Autodesk Inventor part; units mm, degrees
ref_plane "YZ Plane" through (0, 0, 0) normal (1, 0, 0) x (0, 1, 0)
ref_plane "XZ Plane" through (0, 0, 0) normal (0, 1, 0) x (-1, 0, 0)
ref_plane "XY Plane" through (0, 0, 0) normal (0, 0, 1) x (1, 0, 0)
sketch "Sketch1" plane through (0, 0, 0) normal (0, 0, 1) x (1, 0, 0)
  line L0 (-7, 7) -> (7, 7)
  line L1 (7, 7) -> (7, -7)
  line L2 (7, -7) -> (-7, -7)
  line L3 (-7, -7) -> (-7, 7)
  line L4 (-7, 7) -> (7, -7) construction
  line L5 (7, 7) -> (-7, -7) construction
  point P0 (0, 0)
  dimension "d0" = 14
  dimension "d1" = 14
extrude "Extrusion1" add sketch "Sketch1" along normal blind 28
sketch "Sketch2" plane through (7, -7, 0) normal (1, 0, 0) x (0, 0, -1)
  line L0 (-28, 0) -> (-28, 14)
  line L1 (-28, 14) -> (-14, 14)
  line L2 (-14, 14) -> (-14, 0)
  line L3 (-14, 0) -> (-28, 0)
  line L4 (-28, 0) -> (-28, 14)
  point P0 (0, 7)
  dimension "d4" = 14
  dimension "d5" = 14
extrude "Extrusion2" add sketch "Sketch2" along normal blind 14
sketch "Sketch3" plane through (21, -7, 0) normal (1, 0, 0) x (0, 0, -1)
  line L0 (-14, 0) -> (-14, 14)
  line L1 (-14, 14) -> (-28, 14)
  line L2 (-28, 14) -> (-28, 0)
  line L3 (-28, 0) -> (-14, 0)
  line L4 (-28, 14) -> (-14, 14)
  line L5 (-14, 14) -> (-14, 0)
  line L6 (-14, 0) -> (-28, 0)
  line L7 (-28, 0) -> (-28, 14)
  point P0 (0, 7)
  point P1 (-21, 7)
hole "Hole1" at (21, 0, 21) direction (-1, 0, 0) diameter 8 depth 25
sketch "Sketch4" plane through (0, 0, 0) normal (0, 0, -1) x (-1, 0, 0)
  line L0 (7, -7) -> (-7, -7)
  line L1 (7, 7) -> (7, -7)
  line L2 (-7, 7) -> (7, 7)
  line L3 (-7, -7) -> (-7, 7)
  point P0 (0, 0)
  point P1 (0, 0)
sketch "Sketch5" plane through (-7, 7, 0) normal (0, 1, 0) x (1, 0, 0)
  line L0 (14, 0) -> (0, 0)
  line L1 (0, 0) -> (0, -28)
  line L2 (0, -28) -> (28, -28)
  line L3 (28, -14) -> (28, -28)
  line L4 (14, -14) -> (28, -14)
  line L5 (14, 0) -> (14, -14)
  line L6 (14, -14) -> (28, -14)
  line L7 (28, -14) -> (28, -28)
  line L8 (28, -28) -> (14, -28)
  line L9 (14, -28) -> (14, -14)
  circle A0 centre (21, -21) radius 4
  point P0 (7, 0)
  dimension "d23" = 8
extrude "Extrusion3" add sketch "Sketch5" along normal blind 45 contours A0
thread "Thread1"
sketch "Sketch6" plane through (14, 52, 21) normal (0, 1, 0) x (1, 0, 0)
  circle A0 centre (0, 0) radius 4
  point P0 (-14, 21)
hole "Hole3" at (14, 52, 21) direction (0, -1, 0) diameter 6 depth 50 tip angle 118
sketch "Sketch7" plane through (-7, -7, 0) normal (0, -1, 0) x (1, 0, 0)
  line L0 (28, 28) -> (28, 14)
  line L1 (14, 14) -> (28, 14)
  line L2 (28, 28) -> (14, 28)
  line L3 (14, 28) -> (14, 14)
  line L4 (14, 14) -> (28, 14)
  line L5 (28, 14) -> (28, 28)
  circle A0 centre (21, 21) radius 3
  circle A1 centre (21, 21) radius 7
  circle A2 centre (21, 21) radius 4
  circle A3 centre (21, 21) radius 4
  line L6 (21, 21) -> (0, 21)
  line L7 (0, 0) -> (0, 28)
  line L8 (0, 21) -> (0, 34.5)
  line L9 (0, 34.5) -> (0, 21)
  line L10 (0, 21) -> (0, 7.5)
  point P0 (7, 0)
  dimension "d35" = 14
  dimension "d36" = 8
  dimension "d37" = 13.5
  dimension "d38" = 13.5
sketch "Sketch8" plane through (0, 0, 0) normal (0, 0, -1) x (-1, 0, 0)
  line L0 (7, -7) -> (-7, -7)
  line L1 (7, 7) -> (7, -7)
  line L2 (-7, -7) -> (7, -7)
  line L3 (7, -7) -> (7, 7)
  line L4 (7, 7) -> (-7, 7)
  line L5 (-7, 7) -> (-7, -7)
  point P0 (0, 0)
extrude "Extrusion4" cut sketch "Sketch8" against normal blind 7.5
sketch "Sketch9" plane through (0, 0, 28) normal (0, 0, 1) x (1, 0, 0)
  line L0 (-7, 7) -> (21, 7)
  line L1 (-7, 7) -> (7, 7)
  line L2 (7, 7) -> (7, -7)
  line L3 (7, -7) -> (-7, -7)
  line L4 (-7, -7) -> (-7, 7)
  point P0 (0, 0)
  dimension "d41" = 14
  dimension "d42" = 14
extrude "Extrusion5" add sketch "Sketch9" along normal blind 6.5
hole "Hole4" at (0, 0, 0) direction (0, 0, 1) diameter 8 end through all
extrude "Extrusion6" add sketch "Sketch7" along normal blind 14 contours A1
thread "Thread2"
sketch "Sketch10" plane through (14, -7, 21) normal (0, -1, 0) x (1, 0, 0)
  circle A0 centre (0, 0) radius 4
  point P0 (-14, -21)
hole "Hole5" at (14, -7, 21) direction (0, 1, 0) diameter 5 depth 8
properties part number "HUDSON-1-45"
Part model, mm, in its own coordinate system. A direction names the side the tool comes from. Give positions to 0.01 mm unless a question says otherwise; leave off trailing zeros. Write each loop counter-clockwise with the first axis right and the second up, starting at its lowest first coordinate (ties: lowest second). Pieces come first, ordered by that corner, then holes.
1) Cut at C-C on z = 22. State how many separate pieces and enclosed holes the cut face has, then the cut area to 3 significant figures.
Resolved:
separate pieces: 3
enclosed holes: 0
area: 346 mm2
2) Probe L1, parallel to Z at x = 14, y = 20.5; L2, parallel to Z at x = 14, y = -4.85; L3, parallel to Y at x = 0, z = 13.5. List the from-to ranges inside material, lowest first.
Resolved:
L1: z = 17 to 18, 24 to 25
L2: z = 14 to 18.5, 23.5 to 28
L3: y = -7 to -4, 4 to 7
3) Cut at B-B on y = -2. Write the cut outline in (x, z).
Resolved:
outline: (-7, 7.5) - (-3.46, 7.5) - (-3.46, 17.54) - (-4, 17.54) - (-4, 24.46) - (-3.46, 24.46) - (-3.46, 34.5) - (-7, 34.5) - close; (3.46, 7.5) - (7, 7.5) - (7, 14) - (21, 14) - (21, 17.54) - (3.46, 17.54) - close; (3.46, 24.46) - (21, 24.46) - (21, 28) - (7, 28) - (7, 34.5) - (3.46, 34.5) - close
4) Pin check, flat tips, straight feed: pin 1 (10 mm diameter, centred on x = 2, y = 12.5, fed in from +Z); pin 2 (2 mm diameter, centred on y = 34, z = 16.5, fed in from -X); pin 3 (1 mm diameter, centred on x = 9.5, z = 17.5, fed in from +Y); pin 4 (6.5 mm diameter, centred on y = 0, z = 21, fed in from +X). Stop position of each tip, or through.
Resolved:
pin 1: passes through
pin 2: stops at x = 12.06
pin 3: stops at y = 7
pin 4: stops at x = -4
5) Cut at A-A on x = 15. Write the cut outline in (y, z), then the cut area to 3 significant figures.
Resolved:
outline: (-21, 14.07) - (-7, 14.07) - (-7, 14) - (7, 14) - (7, 17.13) - (52, 17.13) - (52, 18.17) - (2.83, 18.17) arc R4 cw to (-3.28, 18.71) - (-7, 18.71) - (-7, 17.13) - (-21, 17.13) - close; (-21, 24.87) - (-7, 24.87) - (-7, 23.29) - (-3.28, 23.29) arc R4 cw to (2.83, 23.83) - (52, 23.83) - (52, 24.87) - (7, 24.87) - (7, 28) - (-7, 28) - (-7, 27.93) - (-21, 27.93) - close
area: 291 mm2
6) Two-plate mould, pull along Z, no slides. Class faces 4 (the face through (-3, 4, 21)), 5 (the face through (12.483, -13.902, 27.834)), 6 (the face through (7, 0, 31)): released by +Z, released by -Z, zero draft, split by the parting line, or undercut.
Resolved:
face 4: undercut
face 5: split by the parting line
face 6: zero draft
7) Cut at D-D on y = -12.5. Write the cut outline in (x, z), then the cut area to 3 significant figures.
Resolved:
outline: circle Ø14 at (14, 21); hole circle Ø8 at (14, 21)
area: 104 mm2
8) Which spindle directions (+Z, -Z, +X, -X, +Y, -Y) get a long thin tool onto all of the face, cutting with end or side? Do faces 1 (the face through (10.35, -2.7, 23.95)), 2 (the face through (16.93, 26.98, 20.35)), 3 (the face through (16, -7, 23)). Say none if no direction does.
Resolved:
face 1: +X
face 2: +Y
face 3: -Y
